For this review, use the dimensioned drawing (mm, ordinates from the lowest corner) and the shaded views. Coordinates: 2 decimals unless noted, no trailing zeros. Write each loop counter-clockwise with the first axis right and the second up, starting at its lowest first coordinate (ties: lowest second). Pieces come first, ordered by that corner, then holes.
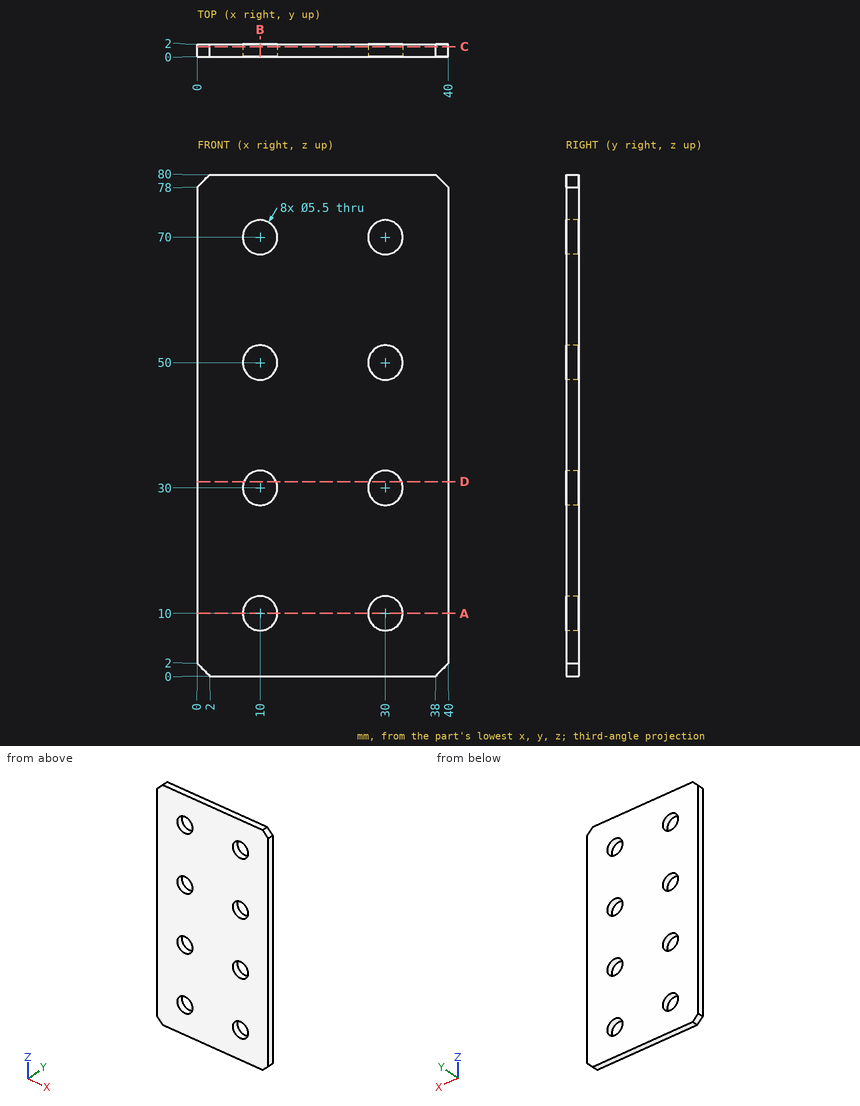
Item 1: For pin 1 (7 mm diameter, centred on x = 30, z = 30, fed in from -Y); pin 2 (4.5 mm diameter, centred on x = 10, z = 70, fed in from +Y), all flat-tipped, find the tip position at first contact; note any pin that passes through.
Solved:
pin 1: stops at y = 0
pin 2: passes through
Item 2: Take a section at A-A, the plane z = 10. Write out the cut boundary in (x, y), plus the area to 3 significant figures.
Solved:
outline: (0, 0) - (7.25, 0) - (7.25, 2) - (0, 2) - close; (12.75, 0) - (27.25, 0) - (27.25, 2) - (12.75, 2) - close; (32.75, 0) - (40, 0) - (40, 2) - (32.75, 2) - close
area: 58.0 mm2
Item 3: Take a section at B-B, the plane x = 10. Write out the cut boundary in (y, z), plus the area to 3 significant figures.
Solved:
outline: (0, 0) - (2, 0) - (2, 7.25) - (0, 7.25) - close; (0, 12.75) - (2, 12.75) - (2, 27.25) - (0, 27.25) - close; (0, 32.75) - (2, 32.75) - (2, 47.25) - (0, 47.25) - close; (0, 52.75) - (2, 52.75) - (2, 67.25) - (0, 67.25) - close; (0, 72.75) - (2, 72.75) - (2, 80) - (0, 80) - close
area: 116 mm2
Item 4: Take a section at C-C, the plane y = 1.6. Count the separate pieces of the cut face and the enclosed holes in it, plus the area to 3 significant figures.
Solved:
separate pieces: 1
enclosed holes: 8
area: 3,000 mm2
Item 5: Take a section at D-D, the plane z = 31. Write out the cut boundary in (x, y).
Solved:
outline: (0, 0) - (7.44, 0) - (7.44, 2) - (0, 2) - close; (12.56, 0) - (27.44, 0) - (27.44, 2) - (12.56, 2) - close; (32.56, 0) - (40, 0) - (40, 2) - (32.56, 2) - close
Item 6: To check wall thickness, follow line 1 along Z through (x, y) = (30, 1); line 2 along X through (y, z) = (1.15, 50); line 3 along Z through (x, y) = (11.5, 0.15). State the ranges of each line that lie inside material, in increasing order.
Solved:
line 1: z = 0 to 7.25, 12.75 to 27.25, 32.75 to 47.25, 52.75 to 67.25, 72.75 to 80
line 2: x = 0 to 7.25, 12.75 to 27.25, 32.75 to 40
line 3: z = 0 to 7.7, 12.3 to 27.7, 32.3 to 47.7, 52.3 to 67.7, 72.3 to 80
